from build123d import *

# Parameters (mm, degrees)
BOSS_EXTRUDE1_DEPTH   = 82.55
SKETCH2_W             = 152.4
SKETCH2_H             = 279.4
CUT_EXTRUDE1_DEPTH    = 242.3
SKETCH3_R             = 25.4
BOSS_EXTRUDE2_DEPTH   = 12.7
SKETCH3_R_2           = 38.1
BOSS_EXTRUDE2_2_DEPTH = 12.7
BOSS_EXTRUDE2_3_DEPTH = 12.7
BOSS_EXTRUDE2_4_DEPTH = 12.7
SKETCH4_R             = 6.35
BOSS_EXTRUDE3_DEPTH   = 76.2


with BuildPart() as part:
    # Sketch1 → Boss-Extrude1 (new body, symmetric)
    with BuildSketch(Plane(origin=(0, 0, 0), x_dir=(0, 0, -1), z_dir=(1, 0, 0))):
        Polygon((0, 0), (228.6, 0), (228.6, 127), (279.4, 127), (279.4, 241.3), (0, 241.3), align=None)
    extrude(amount=BOSS_EXTRUDE1_DEPTH, both=True)

    # Sketch2 → Cut-Extrude1 (cut, through all)
    with BuildSketch(Plane(origin=(0, 241.3, 0), x_dir=(1, 0, 0), z_dir=(0, 1, 0))):
        with Locations((0, 139.7)):
            Rectangle(SKETCH2_W, SKETCH2_H)
    extrude(amount=-CUT_EXTRUDE1_DEPTH, mode=Mode.SUBTRACT)



with BuildPart() as body_2:
    # Sketch3 → Boss-Extrude2 (new body, symmetric)
    with BuildSketch(Plane(origin=(0, 0, 0), x_dir=(0, 0, -1), z_dir=(1, 0, 0))):
        with Locations((161.472166443, 31.75)):
            Circle(SKETCH3_R)
    extrude(amount=BOSS_EXTRUDE2_DEPTH, both=True)


with BuildPart() as body_3:
    # Sketch3 → Boss-Extrude2 2 (new body, symmetric)
    with BuildSketch(Plane(origin=(0, 0, 0), x_dir=(0, 0, -1), z_dir=(1, 0, 0))):
        with Locations((240.017328611, 184.15)):
            Circle(SKETCH3_R_2)
    extrude(amount=BOSS_EXTRUDE2_2_DEPTH, both=True)


with BuildPart() as body_4:
    # Sketch3 → Boss-Extrude2 3 (new body, symmetric)
    with BuildSketch(Plane(origin=(0, 0, 0), x_dir=(0, 0, -1), z_dir=(1, 0, 0))):
        with Locations((69.85, 163.217184297)):
            Circle(SKETCH3_R)
    extrude(amount=BOSS_EXTRUDE2_3_DEPTH, both=True)


with BuildPart() as body_5:
    # Sketch3 → Boss-Extrude2 4 (new body, symmetric)
    with BuildSketch(Plane(origin=(0, 0, 0), x_dir=(0, 0, -1), z_dir=(1, 0, 0))):
        with Locations((99.356812104, 86.120812531)):
            Circle(SKETCH3_R)
    extrude(amount=BOSS_EXTRUDE2_4_DEPTH, both=True)


with BuildPart() as part_1:
    add(part.part)

    add(body_2.part)  # Boss-Extrude3 merges body 2

    add(body_3.part)  # Boss-Extrude3 merges body 3

    add(body_4.part)  # Boss-Extrude3 merges body 4

    add(body_5.part)  # Boss-Extrude3 merges body 5
    # Sketch4 → Boss-Extrude3 (add, symmetric)
    with BuildSketch(Plane(origin=(0, 0, 0), x_dir=(0, 0, -1), z_dir=(1, 0, 0))):
        with Locations((69.85, 163.217184297)):
            Circle(SKETCH4_R)
        with Locations((99.356812104, 86.120812531)):
            Circle(SKETCH4_R)
        with Locations((161.472166443, 31.75)):
            Circle(SKETCH4_R)
        with Locations((240.017328611, 184.15)):
            Circle(SKETCH4_R)
    extrude(amount=BOSS_EXTRUDE3_DEPTH, both=True)


solid = part_1.part
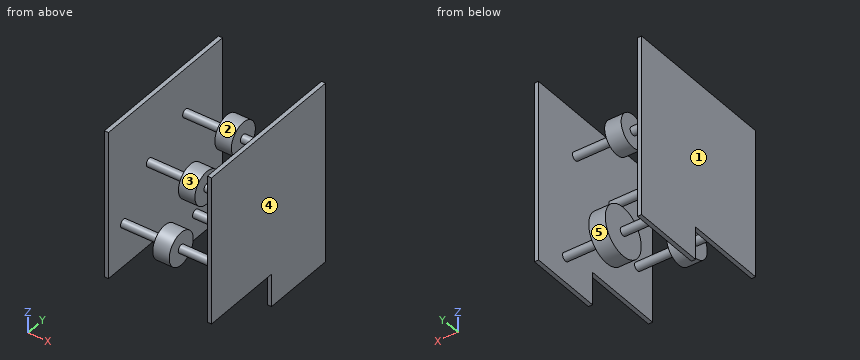
Could you check a few things on this model? Use its own coordinates, in mm. Face numbers are marked on the shaded views. A direction names the side the tool comes from. Give positions to 0.01 mm unless a question says otherwise; leave off trailing zeros. Write each loop counter-clockwise with the first axis right and the second up, starting at its lowest first coordinate (ties: lowest second). Pieces come first, ordered by that corner, then holes. Notation, with made-up numbers: (74, 45.25) - (130, 45.25) arc R13 ccw to (130, 64.25) - close; hole circle Ø4 at (-34, -11.5). An arc over 180 degrees is marked (long way). Use CSV: the item, a comma, the result in double quotes. Start each with the question number.
Item 1: I'm going to push flat-ended pins straight in: pin 1 (7 mm diameter, centred on x = -80, z = -258, fed in from -Y); pin 2 (1.9 mm diameter, centred on x = 79.5, y = 90.5, fed in from -Z); pin 3 (2 mm diameter, centred on x = -9.5, z = -227.5, fed in from -Y). Where does each tip first touch, or does it pass through?
Item 2: I want a section at D-D, the plane z = -79.5. Please give me the cut outline in (x, y).
Item 3: If I drill on line 1 along X through (y, z) = (155, -240); line 2 along X through (y, z) = (128, -214.5); line 3 along Y through (x, z) = (-27.5, -160.5), over which ranges is the centre line in solid material (lowest first)?
Item 4: If we mould it in two halves opening along Z, with no side actions, what happens to the marked faces 1, 2 and 3? For each: pulls with the +Z half, pulls with the -Z half, needs draft (parallel to the pull), parting line crosses it, or undercut.
Item 5: For the marked faces 4 and 5, which set-ups out of +Z, -Z, +X, -X, +Y, -Y let a thin tool reach every point of the face, with its end or its side?
Item 6: I want a section at C-C, the plane y = 212. Please give me the cut outline in (x, z).
Item 7: I want a section at A-A, the plane z = -19. Please give me the cut outline in (x, y).
Item 8: I want a section at B-B, the plane z = -49. Please give me the cut outline in (x, y), then the cut area to 3 significant figures.
Findings:
1,pin 1,"stops at y = 127"
1,pin 2,"stops at z = -228.6"
1,pin 3,"stops at y = 147.83"
2,outline,"(-82.55, 0) - (-76.2, 0) - (-76.2, 241.3) - (-82.55, 241.3) - close; (-12.7, 70.28) - (12.7, 70.28) - (12.7, 101.96) - (-12.7, 101.96) - close; (-12.7, 139.72) - (12.7, 139.72) - (12.7, 186.71) - (-12.7, 186.71) - close; (76.2, 0) - (82.55, 0) - (82.55, 241.3) - (76.2, 241.3) - close"
3,line 1,"x = -82.55 to -76.2, -12.7 to 12.7, 76.2 to 82.55"
3,line 2,"x = -82.55 to -76.2, 76.2 to 82.55"
3,line 3,"y = 25.47 to 38.03"
4,face 1,"needs draft"
4,face 2,"undercut"
4,face 3,"parting line crosses it"
5,face 4,"+Z, -Z, +X, +Y, -Y"
5,face 5,"none"
6,outline,"(-82.55, -279.4) - (-76.2, -279.4) - (-76.2, 0) - (-82.55, 0) - close; (-12.7, -266.02) - (12.7, -266.02) - (12.7, -214.02) - (-12.7, -214.02) - close; (76.2, -279.4) - (82.55, -279.4) - (82.55, 0) - (76.2, 0) - close"
7,outline,"(-82.55, 0) - (-76.2, 0) - (-76.2, 241.3) - (-82.55, 241.3) - close; (76.2, 0) - (82.55, 0) - (82.55, 241.3) - (76.2, 241.3) - close"
8,outline,"(-82.55, 0) - (-76.2, 0) - (-76.2, 241.3) - (-82.55, 241.3) - close; (-12.7, 148.71) - (12.7, 148.71) - (12.7, 177.72) - (-12.7, 177.72) - close; (76.2, 0) - (82.55, 0) - (82.55, 241.3) - (76.2, 241.3) - close"
8,area,"3,800 mm2"
